Source: CAD feature listing. Evaluate the final solid. Frame: model axes, mm. Coordinates: 2 decimals unless noted, no trailing zeros. Write each loop counter-clockwise with the first axis right and the second up, starting at its lowest first coordinate (ties: lowest second). Pieces come first, ordered by that corner, then holes. Notation, with made-up numbers: (77, -25) - (124, -25) arc R20 ccw to (124, 12) - close; hole circle Ø8 at (78, -28). An arc over 180 degrees is marked (long way). One line per question, with ' | ' between items.
Autodesk Inventor part; units mm, degrees
ref_plane "YZ Plane" through (0, 0, 0) normal (1, 0, 0) x (0, 1, 0)
ref_plane "XZ Plane" through (0, 0, 0) normal (0, 1, 0) x (-1, 0, 0)
ref_plane "XY Plane" through (0, 0, 0) normal (0, 0, 1) x (1, 0, 0)
sketch "Esquisse1" plane through (0, 0, 0) normal (0, 1, 0) x (-1, 0, 0)
  line L0 (50, 0) -> (0, 0)
  line L1 (0, 0) -> (0, -82)
  line L2 (0, -82) -> (50, -82)
  line L3 (50, -82) -> (50, 0)
  point P0 (0, 0)
  dimension "d0" = 0
  dimension "d1" = 0
  dimension "d2" = 50
  dimension "d3" = 82
extrude "Extrusion1" add sketch "Esquisse1" along normal blind 10
sketch "Esquisse2" plane through (-50, 0, 0) normal (0, 0, 1) x (1, 0, 0)
  point P0 (50, 0)
sketch "Esquisse3" plane through (0, 0, 0) normal (1, 0, 0) x (0, 0, -1)
  line L0 (10, 5) -> (72, 5)
  line L1 (0, 0) -> (0, 10)
  circle A0 centre (10, 5) radius 2
  circle A1 centre (72, 5) radius 2
  line L2 (0, 10) -> (82, 10)
  dimension "d7" = 62
  dimension "d8" = 10
  dimension "d9" = 4
  dimension "d10" = 4
  dimension "d11" = 5
hole "Perçage1" at (0, 5, -10) at (0, 5, -72) direction (-1, 0, 0) diameter 4 end through all
properties part number "spacermoteur"
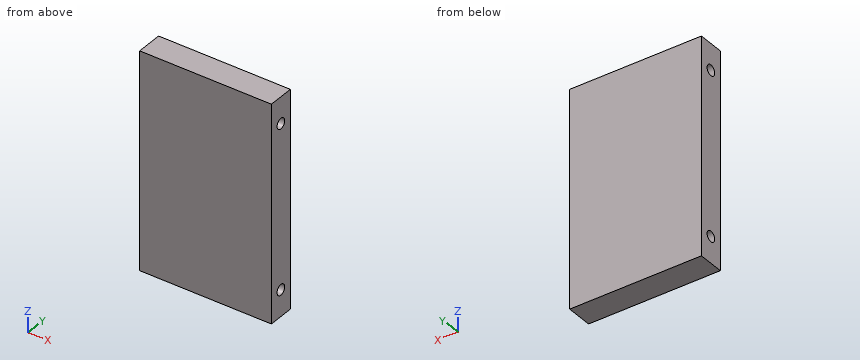
Item 1: Ray query, line 1 along Z through (x, y) = (-28, 5); line 2 along Y through (x, z) = (-13, -72); line 3 along Z through (x, y) = (-12, 5.75). Return the intervals inside material, ascending. Write a range as [from, to].
Check sheet entries:
line 1: [-82, -74], [-70, -12], [-8, 0] | line 2: [0, 3], [7, 10] | line 3: [-82, -73.85], [-70.15, -11.85], [-8.15, 0]
Item 2: Pin query (flat end, axial travel): pin 1 Ø3 at (y, z) = (5, -72) entering from +X. Return the tip coordinate at first contact, or that it passes through.
Check sheet entries:
pin 1: through
Item 3: Cut plane C-C on x = -25.5. Return loops of the section in (y, z), and give its area (3 significant figures).
Check sheet entries:
outline: (0, -82) - (10, -82) - (10, 0) - (0, 0) - close; hole circle Ø4 at (5, -72); hole circle Ø4 at (5, -10) | area: 795 mm²
Item 4: Cut plane B-B on z = -72. Return loops of the section in (x, y).
Check sheet entries:
outline: (-50, 0) - (0, 0) - (0, 3) - (-50, 3) - close; (-50, 7) - (0, 7) - (0, 10) - (-50, 10) - close
Item 5: Cut plane A-A on y = 5. Return loops of the section in (x, z).
Check sheet entries:
outline: (-50, -82) - (0, -82) - (0, -74) - (-50, -74) - close; (-50, -70) - (0, -70) - (0, -12) - (-50, -12) - close; (-50, -8) - (0, -8) - (0, 0) - (-50, 0) - close
